```python
from build123d import *

# Parameters (mm, degrees)
BOSS_EXTRUDE1_DEPTH    = 101.6
BOSS_EXTRUDE2_DEPTH    = 6.35
CUT_EXTRUDE1_START     = 70.369117279
CUT_EXTRUDE1_OUTLINE_R = 6.35
CUT_EXTRUDE1_DEPTH     = 6.35
FLATTEN_BENDS1_START   = 128.994638868
FLATTEN_BENDS1_DEPTH   = 733.419948548
FLATTEN_BENDS1_START_2 = 859.239587416
FLATTEN_BENDS1_2_DEPTH = 3.175
FLATTEN_BENDS1_START_3 = 128.630782005
FLATTEN_BENDS1_3_DEPTH = 2.307819383
FLATTEN_BENDS1_START_4 = 130.938601388
FLATTEN_BENDS1_4_DEPTH = 728.300986028
CHAMFER1_SIZE          = 3.9624


# Read off the part's stored shape, not the designer's step: Cut-Extrude1, Flatten-Bends1
with BuildPart() as part:
    # Sketch11 → Boss-Extrude1 (new, symmetric)
    with BuildSketch(Plane(origin=(0, 0, 0), x_dir=(0, 0, -1), z_dir=(1, 0, 0))):
        Polygon((-57.083945563, 140.613525126), (-50.8, 139.7), (53.975, 860.425), (47.691054437, 861.338525126), align=None)
    extrude(amount=BOSS_EXTRUDE1_DEPTH, both=True)

    # Sketch8 → Boss-Extrude2 (add)
    with BuildSketch(Plane(origin=(101.6, 0, 0), x_dir=(0, 0, -1), z_dir=(1, 0, 0))):
        with BuildLine():
            Line((-130.175, 139.7), (-57.216748776, 139.7))
            Line((-57.216748776, 139.7), (-57.083945563, 140.613525126))
            Line((-57.083945563, 140.613525126), (-50.8, 139.7))
            Line((-50.8, 139.7), (53.975, 860.425))
            Line((53.975, 860.425), (49.2125, 861.117345815))
            Line((49.2125, 861.117345815), (49.2125, 925.5125))
            ThreePointArc((49.2125, 925.5125), (47.352628061, 930.002628061), (42.8625, 931.8625))
            Line((42.8625, 931.8625), (-29.563705158, 931.8625))
            ThreePointArc((-29.563705158, 931.8625), (-40.468229819, 928.432802235), (-47.446326779, 919.378651382))
            Line((-47.446326779, 919.378651382), (-139.7, 668.12987028))
            Line((-139.7, 668.12987028), (-139.7, 660.4))
            Line((-139.7, 660.4), (-130.175, 660.4))
            Line((-130.175, 660.4), (-130.175, 139.7))
        make_face()
    boss_extrude2 = extrude(amount=-BOSS_EXTRUDE2_DEPTH)

    # Mirror1: Boss-Extrude2 across plane
    add(boss_extrude2.mirror(Plane(origin=(0, 0, 0), x_dir=(0, 0, 1), z_dir=(1, 0, 0))))

    # Cut-Extrude1 outline → Cut-Extrude1 (cut)
    with BuildSketch(Plane(origin=(0, 0, 0), x_dir=(1, 0, 0), z_dir=(0, 0.143862224560971, 0.989597726525465)).offset(CUT_EXTRUDE1_START)):
        with Locations((50.8, 638.938601388)):
            Circle(CUT_EXTRUDE1_OUTLINE_R)
        with Locations((50.8, 689.738601388)):
            Circle(CUT_EXTRUDE1_OUTLINE_R)
        with Locations((-50.8, 638.938601388)):
            Circle(CUT_EXTRUDE1_OUTLINE_R)
        with Locations((-50.8, 689.738601388)):
            Circle(CUT_EXTRUDE1_OUTLINE_R)
    extrude(amount=CUT_EXTRUDE1_DEPTH, mode=Mode.SUBTRACT)

    # Flatten-Bends1 outline → Flatten-Bends1 (cut)
    with BuildSketch(Plane(origin=(0, 0, 0), x_dir=(1, 0, 0), z_dir=(0, 0.989597726525465, -0.143862224560971)).offset(FLATTEN_BENDS1_START)):
        with BuildLine():
            ThreePointArc((-101.6, -83.069117279), (-97.880256121, -74.088861158), (-88.9, -70.369117279))
            Line((-88.9, -70.369117279), (-101.6, -70.369117279))
            Line((-101.6, -70.369117279), (-101.6, -83.069117279))
        make_face()
        with BuildLine():
            Line((101.6, -70.369117279), (88.9, -70.369117279))
            ThreePointArc((88.9, -70.369117279), (97.880256121, -74.088861158), (101.6, -83.069117279))
            Line((101.6, -83.069117279), (101.6, -70.369117279))
        make_face()
    extrude(amount=FLATTEN_BENDS1_DEPTH, mode=Mode.SUBTRACT)

    # Flatten-Bends1 2 outline → Flatten-Bends1 2 (cut)
    with BuildSketch(Plane(origin=(0, 0, 0), x_dir=(1, 0, 0), z_dir=(0, 0.989597726525465, -0.143862224560971)).offset(FLATTEN_BENDS1_START_2)):
        with BuildLine():
            Line((-101.6, -83.069117279), (-101.6, -91.05667886))
            Line((-101.6, -91.05667886), (-95.25, -91.05667886))
            Line((-95.25, -91.05667886), (-95.25, -76.719117279))
            Line((-95.25, -76.719117279), (95.25, -76.719117279))
            Line((95.25, -76.719117279), (95.25, -91.05667886))
            Line((95.25, -91.05667886), (101.6, -91.05667886))
            Line((101.6, -91.05667886), (101.6, -83.069117279))
            ThreePointArc((101.6, -83.069117279), (97.880256121, -74.088861158), (88.9, -70.369117279))
            Line((88.9, -70.369117279), (-88.9, -70.369117279))
            ThreePointArc((-88.9, -70.369117279), (-97.880256121, -74.088861158), (-101.6, -83.069117279))
        make_face()
    extrude(amount=FLATTEN_BENDS1_2_DEPTH, mode=Mode.SUBTRACT)

    # Flatten-Bends1 3 outline → Flatten-Bends1 3 (cut)
    with BuildSketch(Plane(origin=(0, 0, 0), x_dir=(1, 0, 0), z_dir=(0, 0.989597726525465, -0.143862224560971)).offset(FLATTEN_BENDS1_START_3)):
        with BuildLine():
            Line((-101.6, -83.069117279), (-101.6, -86.244117279))
            Line((-101.6, -86.244117279), (-95.25, -86.244117279))
            Line((-95.25, -86.244117279), (-95.25, -76.719117279))
            Line((-95.25, -76.719117279), (-99.898522628, -76.719117279))
            ThreePointArc((-99.898522628, -76.719117279), (-101.167257994, -79.782115406), (-101.6, -83.069117279))
        make_face()
        with BuildLine():
            Line((95.25, -76.719117279), (95.25, -86.244117279))
            Line((95.25, -86.244117279), (101.6, -86.244117279))
            Line((101.6, -86.244117279), (101.6, -83.069117279))
            ThreePointArc((101.6, -83.069117279), (101.167257994, -79.782115406), (99.898522628, -76.719117279))
            Line((99.898522628, -76.719117279), (95.25, -76.719117279))
        make_face()
    extrude(amount=FLATTEN_BENDS1_3_DEPTH, mode=Mode.SUBTRACT)

    # Flatten-Bends1 4 outline → Flatten-Bends1 4 (add)
    with BuildSketch(Plane(origin=(0, 0, 0), x_dir=(1, 0, 0), z_dir=(0, 0.989597726525465, -0.143862224560971)).offset(FLATTEN_BENDS1_START_4)):
        with BuildLine():
            Line((-95.25, -76.719117279), (-95.25, -83.069117279))
            ThreePointArc((-95.25, -83.069117279), (-93.390128061, -78.578989218), (-88.9, -76.719117279))
            Line((-88.9, -76.719117279), (-95.25, -76.719117279))
        make_face()
        with BuildLine():
            Line((95.25, -76.719117279), (88.9, -76.719117279))
            ThreePointArc((88.9, -76.719117279), (93.390128061, -78.578989218), (95.25, -83.069117279))
            Line((95.25, -83.069117279), (95.25, -76.719117279))
        make_face()
    extrude(amount=FLATTEN_BENDS1_4_DEPTH)

    # Chamfer1
    chamfer1_edges = [part.edges().sort_by_distance(p)[0] for p in [
        (101.6, 862.826604441, -37.454872482),
        (0, 860.425, -53.975),
        (97.880256121, 860.960130629, -50.293949914),
        (-97.880256121, 860.960130629, -50.293949914),
        (-101.6, 862.826604441, -37.454872482),
    ]]
    chamfer(chamfer1_edges, length=CHAMFER1_SIZE)


solid = part.part
```
Verification items for the finished model (mm, model axes). A direction names the side the tool comes from. Round coordinates to 2 decimals unless told otherwise and drop trailing zeros. Write each loop counter-clockwise with the first axis right and the second up, starting at its lowest first coordinate (ties: lowest second). Pieces come first, ordered by that corner, then holes.
1. Gauge pin test, flat ends, axial feed: P1, Ø5, axis at x = -99.5, y = 903, coming from the -Z side; P2, Ø8, axis at x = -48, y = 489, coming from the +Z side; P3, Ø3, axis at x = 99, z = 134, coming from the -Y side. Record the tip position at first contact, or that the pin passes through.
2. Access from +Z, -Z, +X, -X, +Y, -Y to the whole of each face (thin tool, end or side, straight path). Record for faces 1 (the flat face through (98.47, 795.51, 92.93)), 2 (the flat face through (95.25, 541, 47)).
3. Section check A-A on z = 90. Enter the section's corners in (x, y).
4. Scan lines: L1, parallel to X at y = 466.5, z = 42; L2, parallel to Z at x = -17.5, y = 741.5; L3, parallel to Z at x = 66.5, y = 217. Record each from-to range of solid material in increasing order.
5. Section check B-B on x = -22. Enter the section's corners in (y, z).
6. Draft check along X on faces 3 (the flat face through (1.245, 493.084, -0.573)), 4 (the flat face through (-95.25, 541, 47)), 5 (the flat face through (-101.6, 541, 47)), 6 (the flat face through (101.6, 541, 47)). Enter one of: +X half, -X half, draft (parallel to the pull), parting line (faces both ways), or undercut.
Answer:
1. P1: stops at z = -49.21
1. P2: stops at z = 7.02
1. P3: stops at y = 660.4
2. face 1: +Z, +X, -X, +Y
2. face 2: +Z, +Y
3. outline: (-101.6, 139.7) - (-95.25, 139.7) - (-95.25, 803.49) - (-101.6, 803.49) - close; (95.25, 139.7) - (101.6, 139.7) - (101.6, 803.49) - (95.25, 803.49) - close
4. L1: x = -101.6 to -95.25, 95.25 to 101.6
4. L2: z = -36.69 to -30.27
4. L3: z = 39.56 to 45.98
5. outline: (139.7, 50.8) - (856.5, -53.4) - (861, -50.05) - (861.34, -47.69) - (140.61, 57.08) - close
6. face 3: draft
6. face 4: undercut
6. face 5: -X half
6. face 6: +X half
